from build123d import *

# Parameters (mm, degrees)
BOSS_EXTRUDE1_DEPTH      = 0.405
FILLET1_R                = 1.12
CHAMFER1_SIZE            = 0.5
SKETCH2_R                = 1.1
CUT_EXTRUDE1_DEPTH       = 16.574075414
BOSS_EXTRUDE2_DEPTH      = 0.5
BOSS_EXTRUDE2_DEPTH_BACK = 5.1
SKETCH4_W                = 2.941717286
SKETCH4_H                = 0.549853698
BOSS_EXTRUDE3_DEPTH      = 0.05
BOSS_EXTRUDE4_DEPTH      = 0.525
SKETCH6_R                = 0.577649515
CUT_EXTRUDE2_DEPTH       = 17.26947218
SKETCH7_W                = 50.5
SKETCH7_H                = 23.21
BOSS_EXTRUDE5_DEPTH      = 0.81
FILLET2_R                = 1.12
SKETCH8_W                = 6.401014247
SKETCH8_H                = 5.029368337
SKETCH8_W_2              = 5.38498024
SKETCH8_H_2              = 4.114937731
SKETCH8_W_3              = 3.96253263
SKETCH8_H_3              = 2.617558371
BOSS_EXTRUDE6_DEPTH      = 0.75
BOSS_EXTRUDE7_DEPTH      = 7.5
SKETCH10_W               = 0.132636096
SKETCH10_H               = 11.074362277
CUT_EXTRUDE3_DEPTH       = 6.8
SKETCH11_R               = 1.123282604
SKETCH11_R_2             = 1.136386451
CUT_EXTRUDE4_DEPTH       = 0.3


with BuildPart() as part:
    # Sketch1 → Boss-Extrude1 (new, symmetric)
    with BuildSketch(Plane(origin=(0, 0, 0), x_dir=(1, 0, 0), z_dir=(0, 1, 0))):
        Polygon((-13.55, 7.635), (11.83, 7.635), (11.83, 3.675), (13.55, 2.295), (13.55, -2.295), (11.83, -3.675), (11.83, -7.635), (-13.55, -7.635), align=None)
    extrude(amount=BOSS_EXTRUDE1_DEPTH, both=True)

    # Fillet1
    fillet1_edges = [part.edges().sort_by_distance(p)[0] for p in [
        (-13.55, 0, -7.635),
        (-13.55, 0, 7.635),
    ]]
    fillet(fillet1_edges, radius=FILLET1_R)

    # Chamfer1
    chamfer1_edges = [part.edges().sort_by_distance(p)[0] for p in [
        (11.83, 0, -7.635),
        (11.83, 0, 7.635),
    ]]
    chamfer(chamfer1_edges, length=CHAMFER1_SIZE)

    # Sketch2 → Cut-Extrude1 (cut, through all)
    with BuildSketch(Plane(origin=(0, 0.405, 0), x_dir=(1, 0, 0), z_dir=(0, 1, 0))):
        with Locations(Location((9.57, 5.74, 0), (0, 0, 270))):
            Circle(SKETCH2_R)
        with Locations(Location((9.57, -5.74, 0), (0, 0, 270))):
            Circle(SKETCH2_R)
    extrude(amount=-CUT_EXTRUDE1_DEPTH, mode=Mode.SUBTRACT)

    # Sketch4 → Boss-Extrude3 (add)
    with BuildSketch(Plane(origin=(0, 0.405, 0), x_dir=(1, 0, 0), z_dir=(0, 1, 0))):
        with Locations((-10.930908088, 4.275112504)):
            Rectangle(SKETCH4_W, SKETCH4_H)
        with Locations((-10.930908088, -4.275112504)):
            Rectangle(SKETCH4_W, SKETCH4_H)
    extrude(amount=BOSS_EXTRUDE3_DEPTH)



with BuildPart() as body_2:
    # Sketch3 → Boss-Extrude2 (new, two sides: drawn at the far end of the back side and taken through both)
    with BuildSketch(Plane.ZY.offset(13.55).offset(-BOSS_EXTRUDE2_DEPTH_BACK)):
        Polygon((-3.91, 1.655), (-2.42, 0.455), (2.42, 0.455), (3.91, 1.655), (3.91, 2.505), (2.42, 3.405), (-2.42, 3.405), (-3.91, 2.505), align=None)
    extrude(amount=BOSS_EXTRUDE2_DEPTH + BOSS_EXTRUDE2_DEPTH_BACK)


with BuildPart() as part_1:
    add(part.part)

    add(body_2.part)  # Boss-Extrude4 merges body 2
    # Sketch5 → Boss-Extrude4 (add, symmetric)
    with BuildSketch(Plane(origin=(-11, 0, 0), x_dir=(0, 0, -1), z_dir=(1, 0, 0))):
        Polygon((4.325381098, 0.455), (4.325381098, 0.509426612), (4.162105788, 0.509426612), (3.964358919, 1.644096311), (3.498388432, 1.644096311), (3.498388432, 1.44259556), (3.964358919, 1.44259556), (4.136474144, 0.455), align=None)
        Polygon((-4.136474144, 0.455), (-4.325381098, 0.455), (-4.325381098, 0.509426612), (-4.162105788, 0.509426612), (-3.964358919, 1.644096311), (-3.498388432, 1.644096311), (-3.498388432, 1.44259556), (-3.964358919, 1.44259556), align=None)
    extrude(amount=BOSS_EXTRUDE4_DEPTH, both=True)

    # Sketch6 → Cut-Extrude2 (cut, through all)
    with BuildSketch(Plane(origin=(0, 0.405, 0), x_dir=(1, 0, 0), z_dir=(0, 1, 0))):
        with Locations(Location((-5.985172419, 5.913658107, 0), (0, 0, 270))):
            Circle(SKETCH6_R)
        with Locations(Location((-3.485172419, 5.913658107, 0), (0, 0, 270))):
            Circle(SKETCH6_R)
        with Locations(Location((-0.985172419, 5.913658107, 0), (0, 0, 270))):
            Circle(SKETCH6_R)
        with Locations(Location((1.514827581, 5.913658107, 0), (0, 0, 270))):
            Circle(SKETCH6_R)
        with Locations(Location((4.014827581, 5.913658107, 0), (0, 0, 270))):
            Circle(SKETCH6_R)
        with Locations(Location((4.014827581, -5.913658107, 0), (0, 0, 90))):
            Circle(SKETCH6_R)
        with Locations(Location((1.514827581, -5.913658107, 0), (0, 0, 90))):
            Circle(SKETCH6_R)
        with Locations(Location((-0.985172419, -5.913658107, 0), (0, 0, 90))):
            Circle(SKETCH6_R)
        with Locations(Location((-3.485172419, -5.913658107, 0), (0, 0, 90))):
            Circle(SKETCH6_R)
        with Locations(Location((-5.985172419, -5.913658107, 0), (0, 0, 90))):
            Circle(SKETCH6_R)
    extrude(amount=-CUT_EXTRUDE2_DEPTH, mode=Mode.SUBTRACT)

    # Sketch7 → Boss-Extrude5 (add)
    with BuildSketch(Plane(origin=(0, 0.405, 0), x_dir=(1, 0, 0), z_dir=(0, 1, 0))):
        with Locations((11.7, 0)):
            Rectangle(SKETCH7_W, SKETCH7_H)
    extrude(amount=-BOSS_EXTRUDE5_DEPTH)

    # Fillet2
    fillet2_edges = [part_1.edges().sort_by_distance(p)[0] for p in [
        (-13.55, 0, 11.605),
        (-13.55, 0, -11.605),
        (36.95, 0, -11.605),
        (36.95, 0, 11.605),
    ]]
    fillet(fillet2_edges, radius=FILLET2_R)

    # Sketch8 → Boss-Extrude6 (add)
    with BuildSketch(Plane(origin=(0, 0.405, 0), x_dir=(1, 0, 0), z_dir=(0, 1, 0))):
        with Locations((0.273625917, 0.73916626)):
            Rectangle(SKETCH8_W, SKETCH8_H)
        with Locations((13.482068015, -0.784884752)):
            Rectangle(SKETCH8_W_2, SKETCH8_H_2)
        with Locations((24.8108472, 1.945071243)):
            Rectangle(SKETCH8_W_3, SKETCH8_H_3)
    extrude(amount=BOSS_EXTRUDE6_DEPTH)

    # Sketch9 → Boss-Extrude7 (add, symmetric)
    with BuildSketch(Plane.XY):
        Polygon((37.95, 0.405), (37.95, 5.305), (36.25, 9.005), (32.85, 9.005), (31.15, 5.305), (31.15, 0.405), align=None)
    extrude(amount=BOSS_EXTRUDE7_DEPTH, both=True)

    # Sketch10 → Cut-Extrude3 (cut)
    with BuildSketch(Plane(origin=(37.95, 0, 0), x_dir=(0, 0, -1), z_dir=(1, 0, 0))):
        with Locations((0, 5.942181138)):
            Rectangle(SKETCH10_W, SKETCH10_H)
    extrude(amount=-CUT_EXTRUDE3_DEPTH, mode=Mode.SUBTRACT)

    # Sketch11 → Cut-Extrude4 (cut)
    with BuildSketch(Plane(origin=(0, 9.005, 0), x_dir=(1, 0, 0), z_dir=(0, 1, 0))):
        with Locations(Location((34.55, 5.910055159, 0), (0, 0, 270))):
            Circle(SKETCH11_R)
        with Locations(Location((34.55, 2.205678961, 0), (0, 0, 270))):
            Circle(SKETCH11_R_2)
        with Locations(Location((34.55, -2.205678961, 0), (0, 0, 90))):
            Circle(SKETCH11_R_2)
        with Locations(Location((34.55, -5.910055159, 0), (0, 0, 90))):
            Circle(SKETCH11_R)
    extrude(amount=-CUT_EXTRUDE4_DEPTH, mode=Mode.SUBTRACT)


solid = part_1.part
For this review, take the finished solid that the model builds, in its own axes (mm). A direction names the side the tool comes from. Coordinates: 2 decimals unless noted, no trailing zeros. Loops run counter-clockwise (first coordinate to the right, second up) from the corner with the lowest first, then second, coordinate; pieces in that order, holes last. Notation, with made-up numbers: (30.5, 37) - (67.5, 37) arc R27 ccw to (67.5, 53) - close; hole circle Ø10 at (19.25, 33.25). An arc over 180 degrees is marked (long way). Return JSON: item names as keys, results as strings.
Item 1: Take a section at A-A (y = 4). Give the boundary of the cut face in (x, z).
Determined:
{"outline": "(31.15, -7.5) - (37.95, -7.5) - (37.95, -0.07) - (31.15, -0.07) - close; (31.15, 0.07) - (37.95, 0.07) - (37.95, 7.5) - (31.15, 7.5) - close"}
Item 2: Insertion check: pin 1 (4 mm diameter, centred on x = 3.5, z = 7.5, fed in from +Y) (3 decimals); pin 2 (4 mm diameter, centred on y = 6.5, z = -3, fed in from -X); pin 3 (4 mm diameter, centred on x = 1.5, y = 5, fed in from -Z); pin 4 (2 mm diameter, centred on x = 16, z = 0, fed in from +Y) (3 decimals). Each pin has a flat end and moves straight along its axis. Give the tip position at first contact, or say it passes through.
Determined:
{"pin 1": "stops at y = 0.405", "pin 2": "stops at x = 31.15", "pin 3": "passes through", "pin 4": "stops at y = 1.155"}
Item 3: For line 1 (X direction, y = 2, z = 3.25); line 2 (Y direction, x = 24.5, z = 6) (3 decimals); line 3 (X direction, y = 2, z = 6.5), list the stretches that pass through material, from the lowest coordinate up.
Determined:
{"line 1": "x = -14.05 to -8.45, 31.15 to 37.95", "line 2": "y = -0.405 to 0.405", "line 3": "x = 31.15 to 37.95"}
Item 4: Take a section at B-B (x = 34.55). Give the boundary of the cut face in (y, z) (3 decimals), then the cut area to 3 significant figures.
Determined:
{"outline": "(-0.405, -11.605) - (0.405, -11.605) - (0.405, -7.5) - (9.005, -7.5) - (9.005, -7.033) - (8.705, -7.033) - (8.705, -4.787) - (9.005, -4.787) - (9.005, -3.342) - (8.705, -3.342) - (8.705, -1.069) - (9.005, -1.069) - (9.005, -0.066) - (0.405, -0.066) - (0.405, 0.066) - (9.005, 0.066) - (9.005, 1.069) - (8.705, 1.069) - (8.705, 3.342) - (9.005, 3.342) - (9.005, 4.787) - (8.705, 4.787) - (8.705, 7.033) - (9.005, 7.033) - (9.005, 7.5) - (0.405, 7.5) - (0.405, 11.605) - (-0.405, 11.605) - close", "area": "144 mm2"}
Item 5: Take a section at C-C (x = 13.5). Give the boundary of the cut face in (y, z) (3 decimals), then the cut area to 3 significant figures.
Determined:
{"outline": "(-0.405, -11.605) - (0.405, -11.605) - (0.405, -1.273) - (1.155, -1.273) - (1.155, 2.842) - (0.405, 2.842) - (0.405, 11.605) - (-0.405, 11.605) - close", "area": "21.9 mm2"}
Item 6: Mouldability with a two-part tool opening along Z and no side actions: class faces 1 (the cylindrical face through (-13.2, 0, -11.3)), 2 (the cylindrical face through (-13.2, 0, 11.3)), 3 (the flat face through (-11.211, 1.047, 3.155)) as pulls with the +Z half, pulls with the -Z half, needs draft (parallel to the pull), parting line crosses it, or undercut.
Determined:
{"face 1": "pulls with the -Z half", "face 2": "pulls with the +Z half", "face 3": "undercut"}
Item 7: Take a section at D-D (x = 22). Give the boundary of the cut face in (y, z) (3 decimals), then the cut area to 3 significant figures.
Determined:
{"outline": "(-0.405, -11.605) - (0.405, -11.605) - (0.405, 11.605) - (-0.405, 11.605) - close", "area": "18.8 mm2"}
Item 8: For faces 4 (the flat face through (-11.211, 2.949, 3.175)), 5 (the flat face through (37.4, 0.405, 3.8)), 6 (the flat face through (35, 8.705, -6)), list the 3-axis set-ups (+Z, -Z, +X, -X, +Y, -Y) from which the entire face can be reached by the end or side of a thin tool; tool diameter is ignored.
Determined:
{"face 4": "+Z, -X, +Y", "face 5": "+Z, -Z, +X, -Y", "face 6": "+Y"}
